from build123d import *

# Parameters (mm, degrees)
SKETCH_1_R          = 4
EXTRUDE_1_DEPTH     = 3
EXTRUDE_1_2_DEPTH   = 3
SKETCH_2_W          = 4
SKETCH_2_H          = 22
EXTRUDE_2_DEPTH     = 3
FILLET_1_R          = 3
SKETCH_3_R          = 1.75
CUT_EXTRUDE_1_DEPTH = 3


with BuildPart() as part:
    # Sketch 1 → Extrude 1 (new body)
    with BuildSketch(Plane(origin=(0, 0, 0), x_dir=(1, 0, 0), z_dir=(0, 1, 0))):
        with Locations(Location((0, 0, 0), (0, 0, 270))):
            Circle(SKETCH_1_R)
    extrude(amount=EXTRUDE_1_DEPTH)



with BuildPart() as body_2:
    # Sketch 1 → Extrude 1 2 (new body)
    with BuildSketch(Plane(origin=(0, 0, 0), x_dir=(1, 0, 0), z_dir=(0, 1, 0))):
        with Locations(Location((0, 22, 0), (0, 0, 270))):
            Circle(SKETCH_1_R)
    extrude(amount=EXTRUDE_1_2_DEPTH)


with BuildPart() as part_1:
    add(part.part)

    add(body_2.part)  # Extrude 2 merges body 2
    # Sketch 2 → Extrude 2 (add)
    with BuildSketch(Plane(origin=(0, 3, 0), x_dir=(1, 0, 0), z_dir=(0, 1, 0))):
        with Locations((0, 11)):
            Rectangle(SKETCH_2_W, SKETCH_2_H)
    extrude(amount=-EXTRUDE_2_DEPTH)

    # Fillet 1
    fillet_1_edges = [part_1.edges().sort_by_distance(p)[0] for p in [
        (2, 1.5, -3.464101615),
        (-2, 1.5, -3.464101615),
        (-2, 1.5, -18.535898385),
        (2, 1.5, -18.535898385),
    ]]
    fillet(fillet_1_edges, radius=FILLET_1_R)

    # Sketch 3 → Cut-Extrude 1 (cut)
    with BuildSketch(Plane(origin=(0, 3, 0), x_dir=(1, 0, 0), z_dir=(0, 1, 0))):
        with Locations(Location((0, 22, 0), (0, 0, 270))):
            Circle(SKETCH_3_R)
        with Locations(Location((0, 0, 0), (0, 0, 270))):
            Circle(SKETCH_3_R)
    extrude(amount=-CUT_EXTRUDE_1_DEPTH, mode=Mode.SUBTRACT)


solid = part_1.part
Part model, mm, in its own coordinate system. A direction names the side the tool comes from. Give positions to 0.01 mm unless a question says otherwise; leave off trailing zeros. Loops run counter-clockwise (first coordinate to the right, second up) from the corner with the lowest first, then second, coordinate; pieces in that order, holes last. Notation, with made-up numbers: M 22,30 L 49,30 A16 ccw 49,48 Z; hole C 19.25,59 d8. An arc over 180 degrees is marked long. Put each result on its own line as item: value. Start each with the question number.
1) Pull direction Z, two halves, no side cores. Call faces 1 (the cylindrical face through (-2.216, 1.479, -18.22)), 2 (the cylindrical face through (0, 1, 4)), 3 (the flat face through (0, 3, -11)): +Z half, -Z half, draft (parallel to the pull), parting line (faces both ways), or undercut.
2) Saw through at B-B (y = 1.45). List the corners of the cut face in (x, z).
3) Saw through at A-A (x = 0). List the corners of the cut face in (y, z), then the cut area to 3 significant figures.
4) 3-axis set-ups, long thin cutter, end or side, ignore diameter. For faces 4 (the flat face through (-2, 2, -11)), 5 (the flat face through (0, 0, -11)), 6 (the flat face through (2, 2, -11)): which of +Z, -Z, +X, -X, +Y, -Y reach the whole face in a straight line?
5) Saw through at C-C (z = 0). List the corners of the cut face in (x, y).
6) Saw through at D-D (x = 2.5). List the corners of the cut face in (y, z), then the cut area to 3 significant figures.
7) Flat gauge pins, fed straight in: pin 1 (3 mm diameter, centred on x = 0, z = -22, fed in from +Y); pin 2 (1.5 mm diameter, centred on y = 1, z = -3.5, fed in from -X); pin 3 (1 mm diameter, centred on x = -2, y = 0.5, fed in from +Z); pin 4 (1.5 mm diameter, centred on y = 2.5, z = -9.5, fed in from -X). Where does each tip first touch, or does it go through?
8) Probe probe 1 along X at (y, z) = (1.65, -22); probe 2 along X at (y, z) = (2.9, -10); probe 3 along Z at (x, y) = (3, 2.85). List the from-to ranges inside material, lowest first.
Numbers:
1. face 1: undercut
1. face 2: undercut
1. face 3: draft
2. outline: M -2.86,-19.2 A4 ccw long 2.86,-19.2 A3 cw 2,-17.1 L 2,-4.9 A3 cw 2.86,-2.8 A4 ccw long -2.86,-2.8 A3 cw -2,-4.9 L -2,-17.1 A3 cw Z; hole C 0,-22 d3.5; hole C 0,0 d3.5
3. outline: M 0,-26 L 3,-26 L 3,-23.75 L 0,-23.75 Z; M 0,-20.25 L 3,-20.25 L 3,-1.75 L 0,-1.75 Z; M 0,1.75 L 3,1.75 L 3,4 L 0,4 Z
3. area: 69.0 mm^2
4. face 4: -X, +Y, -Y
4. face 5: +Z, -Z, +X, -X, -Y
4. face 6: +X, +Y, -Y
5. outline: M -4,0 L -1.75,0 L -1.75,3 L -4,3 Z; M 1.75,0 L 4,0 L 4,3 L 1.75,3 Z
6. outline: M 0,-25.12 L 3,-25.12 L 3,-18.76 L 0,-18.76 Z; M 0,-3.24 L 3,-3.24 L 3,3.12 L 0,3.12 Z
6. area: 38.2 mm^2
7. pin 1: through
7. pin 2: x = -2.9
7. pin 3: z = 3.71
7. pin 4: x = -2
8. probe 1: -4 to -1.75, 1.75 to 4
8. probe 2: -2 to 2
8. probe 3: -24.65 to -19.35, -2.65 to 2.65
